Check sheet for the modelled part. Datum: model origin and axes. Units: mm. A direction names the side the tool comes from. Give positions to 0.01 mm unless a question says otherwise; leave off trailing zeros. Loops run counter-clockwise (first coordinate to the right, second up) from the corner with the lowest first, then second, coordinate; pieces in that order, holes last.
Autodesk Inventor part; units mm, degrees
ref_plane "Work Plane1" through (2.4, 0, 0) normal (1, 0, 0) x (0, 0, -1)
ref_plane "YZ Plane" through (0, 0, 0) normal (1, 0, 0) x (0, 1, 0)
ref_plane "XZ Plane" through (0, 0, 0) normal (0, 1, 0) x (-1, 0, 0)
sketch "Sketch1" plane through (0, 0, 0) normal (1, 0, 0) x (0, 1, 0)
  circle A0 centre (0, 0) radius 17
  circle A1 centre (0, 0) radius 14
  dimension "d0" = 34
  dimension "d1" = 28
extrude "Extrusion1" add sketch "Sketch1" along normal blind 0.4 contours A1
ref_plane "Work Plane1" through (2.4, 0, 0) normal (1, 0, 0) x (0, 0, -1)
sketch "Sketch2" plane through (2.4, 0, 0) normal (1, 0, 0) x (0, 0, -1)
  circle A0 centre (0, 0) radius 17
  dimension "d5" = 34
sketch "Sketch3" plane through (0, 0, 0) normal (0, 1, 0) x (-1, 0, 0)
  line L0 (-2.4, 17) -> (-2.4, -17)
  line L1 (0, 14) -> (0, -14)
  line L2 (0, 14) -> (-2.4, 17)
  line L3 (-0.4, 14) -> (-0.4, -14)
  line L4 (-0.4, 14) -> (-2.4, 16.5)
  line L5 (-0.4, 0) -> (-1.3096, 0)
  line L6 (0, 14) -> (-0.4, 14)
  line L7 (-2.4, 16.5) -> (-2.4, 17)
  point P0 (0, 0)
revolve "Revolution1" add sketch "Sketch3" angle 360 about axis through (0.4, 0, 0) along (1, 0, 0)
sketch "Sketch4" plane through (0, 0, 0) normal (-1, 0, 0) x (0, 0, 1)
  circle A0 centre (0, 0) radius 14
  circle A1 centre (0, 0) radius 4.5
  dimension "d7" = 9
extrude "Extrusion2" add sketch "Sketch4" along normal blind 0.6 contours A1
fillet "Fillet1" radius 2 1 edges at (0, 0, -4.5)
sketch "Sketch5" plane through (-0.6, 0, 0) normal (-1, 0, 0) x (0, 0, 1)
  circle A0 centre (0, 0) radius 4.5
  circle A1 centre (0, 0) radius 1
  dimension "d11" = 2
extrude "Extrusion3" add sketch "Sketch5" along normal blind 3 contours A1
sketch "Sketch6" plane through (0.4, 0, 0) normal (1, 0, 0) x (0, 0, -1)
  circle A0 centre (0, 0) radius 14
  circle A1 centre (0, 0) radius 1.35
  dimension "d14" = 2.7
extrude "Extrusion4" add sketch "Sketch6" along normal blind 7.5 contours A1
sketch "Sketch7" plane through (7.9, 0, 0) normal (1, 0, 0) x (0, 0, -1)
  circle A0 centre (0, 0) radius 1
  circle A1 centre (0, 0) radius 1.5
  dimension "d17" = 3
extrude "Extrusion5" add sketch "Sketch7" along normal blind 0.14 contours A0 | A1
sketch "Sketch8" plane through (8.04, 0, 0) normal (1, 0, 0) x (0, 0, -1)
  circle A0 centre (0, 0) radius 1.5
  circle A1 centre (0, 0) radius 1
  dimension "d20" = 2
extrude "Extrusion6" add sketch "Sketch8" along normal blind 11.86 contours A1
chamfer "Chamfer1" distance 0.5 angle 45 1 edges at (8.04, 0, 1)
sketch "Sketch9" plane through (0, 0, 0) normal (0, 0, 1) x (1, 0, 0)
  line L0 (19.9, -1) -> (19.9, 1)
  line L1 (19.9, -0.5) -> (14.9, -1)
  line L2 (8.54, -1) -> (19.9, -1)
  line L3 (19.9, -0.5) -> (19.9, -1)
  line L4 (19.9, -1) -> (15, -1)
  line L5 (23, 0) -> (21.1668, 0)
  point P0 (0, 0)
  dimension "d26" = 0.5
  dimension "d27" = 5
revolve "Revolution2" cut sketch "Sketch9" angle 360 about axis through (23, 0, 0) along (-1, 0, 0)
sketch "Sketch10" plane through (19.9, 0, 0) normal (1, 0, 0) x (0, 0, -1)
  circle A0 centre (0, 0) radius 0.5
  circle A1 centre (0, 0) radius 0.4
  dimension "d29" = 0.8
extrude "Extrusion7" cut sketch "Sketch10" against normal blind 0.1 contours A1
fillet "Fillet2" radius 0.1 1 edges at (19.8, 0, 0.4)
sketch "Sketch11" plane through (-0.6, 0, 0) normal (-1, 0, 0) x (0, 0, 1)
  circle A0 centre (0, 0) radius 1
  circle A1 centre (0, 0) radius 4.5
  circle A2 centre (0, 0) radius 3.25
  dimension "d33" = 6.5
extrude "Extrusion8" add sketch "Sketch11" along normal blind 0.1 contours A2
fillet "Fillet3" radius 0.1 1 edges at (-0.6, 0, -3.25)
properties part number "rubber replica"
(1) Release check for a two-part mould opening along X. For faces 3 (the face through (-3.6, 0, 0)), 4 (the face through (4.1, 1.32, 0.29)), 5 (the face through (2.4, -2.6, -16.45)), 6 (the face through (-2, 1, 0)) record: pulls with the +X half, pulls with the -X half, needs draft (parallel to the pull), parting line crosses it, or undercut.
(2) Section check B-B on x = 3. Record the boundary of the cut face in (y, z).
(3) Gauge pin test, flat ends, axial feed: pin 1 Ø4.5 at (y, z) = (2, 0.5) entering from -X; pin 2 Ø12 at (x, y) = (2.5, 7) entering from -Z; pin 3 Ø0.5 at (y, z) = (0, 0) entering from +X; pin 4 Ø10 at (y, z) = (6.5, -5) entering from +X. Record the tip position at first contact, or that the pin passes through.
(4) Material ranges on line 1 (X direction, y = -2.5, z = 2); line 2 (X direction, y = 9, z = -4.5); line 3 (Z direction, x = 2, y = 4.5), recorded low to high.
(5) Access from +Z, -Z, +X, -X, +Y, -Y to the whole of each face (thin tool, end or side, straight path). Record for faces 1 (the face through (12, 1, 0)), 2 (the face through (0, 3, -6)).
(6) Section check A-A on x = 13. Record the boundary of the cut face in (y, z), plus the area to 3 significant figures.
Computed values:
1. face 3: pulls with the -X half
1. face 4: undercut
1. face 5: pulls with the +X half
1. face 6: needs draft
2. outline: circle Ø2.7 at (0, 0)
3. pin 1: stops at x = -3.6
3. pin 2: stops at z = -16.97
3. pin 3: stops at x = 19.8
3. pin 4: stops at x = 0.4
4. line 1: x = -0.7 to 0.4
4. line 2: x = 0 to 0.4
4. line 3: z = -15.87 to -15.35, 15.35 to 15.87
5. face 1: +X
5. face 2: -X
6. outline: circle Ø2 at (0, 0)
6. area: 3.14 mm2
